Design review of the part built by this model. Coordinates are the model's own, in mm. A direction names the side the tool comes from. Round coordinates to 2 decimals unless told otherwise and drop trailing zeros. Loops run counter-clockwise (first coordinate to the right, second up) from the corner with the lowest first, then second, coordinate; pieces in that order, holes last. Notation, with made-up numbers: (60.5, 49) -> (99.5, 49) arc R19 cw to (99.5, 84) -> close; hole circle Ø11 at (52, 19). An arc over 180 degrees is marked (long way). Answer as CSV lines item,"result". Start each with the question number.
(1) Take a section at A-A, the plane z = -22.75. Write out the cut boundary in (x, y), and give its area (4 significant figures).
(2) For P1, Ø1.5, axis at x = 20.5, y = 1.5, coming from the -Z side; P2, Ø4, axis at x = 0, z = -4.5, coming from the +Y side; P3, Ø1, axis at y = 1.5, z = -71.5, coming from the -X side; P4, Ø0.6, axis at y = 1, z = -71, coming from the +X side, all flat-tipped, find the tip position at first contact; note any pin that passes through.
(3) Machinability: for faces 4 (the face through (21, 2, -70.5)), 5 (the face through (-10, 2, -2)), 6 (the face through (3.671, 1.521, -30.498)), 7 (the face through (-10, 2, -71)), which of the approach directions +Z, -Z, +X, -X, +Y, -Y give a long, thin tool a straight path to every point of the face, cutting with its end or side? Answer none if there is none.
(4) Take a section at D-D, the plane y = 2.45. State how many separate pieces and enclosed holes the cut face has, and give its area (3 significant figures).
(5) Take a section at C-C, the plane z = -36.75. Write out the cut boundary in (x, y).
(6) Take a section at B-B, the plane x = -28.5. Write out the cut boundary in (y, z).
(7) Draft analysis for pull direction X (two halves, no side actions). For faces 1 (the face through (10, 2, -2)), 2 (the face through (0.222, 1.521, -41.795)), 3 (the face through (21, 2, -3)), state which applies: +X half, -X half, draft (parallel to the pull), parting line (faces both ways), or undercut.
(8) To check wall thickness, follow line 1 (X direction, y = 1.15, z = -36.75); line 2 (X direction, y = 0.5, z = -41); line 3 (X direction, y = 2.2, z = -22.75). State the ranges of each line that lie inside material, in increasing order. Write a range as from..to.
from build123d import *

# Parameters (mm, degrees)
BOSS_EXTRUDE1_DEPTH   = 3
CROQUIS13_W           = 23
CROQUIS13_H           = 3
CORTAR_EXTRUIR3_DEPTH = 81.624127902
CUT_EXTRUDE1_REACH    = 82.624
SKETCH3_R             = 1.2
SKETCH3_R_2           = 5.05
SKETCH3_R_3           = 1.75
CHAFL_N3_SIZE         = 1
CORTAR_EXTRUIR2_DEPTH = 81.624127902


with BuildPart() as part:
    # Sketch1 → Boss-Extrude1 (new body)
    with BuildSketch(Plane(origin=(0, 0, 0), x_dir=(1, 0, 0), z_dir=(0, 1, 0))):
        Polygon((-33, 27.237606732), (-33, 0), (33, 0), (33, 73.5), (-33, 73.5), align=None)
    extrude(amount=BOSS_EXTRUDE1_DEPTH)

    # Croquis13 → Cortar-Extruir3 (cut, through all)
    with BuildSketch(Plane(origin=(0, 3, 0), x_dir=(1, 0, 0), z_dir=(0, 1, 0))):
        with Locations((-21.5, 72)):
            Rectangle(CROQUIS13_W, CROQUIS13_H)
        with Locations((21.5, 72)):
            Rectangle(CROQUIS13_W, CROQUIS13_H)
        with Locations((-21.5, 1.5)):
            Rectangle(CROQUIS13_W, CROQUIS13_H)
        with Locations((21.5, 1.5)):
            Rectangle(CROQUIS13_W, CROQUIS13_H)
    extrude(amount=-CORTAR_EXTRUIR3_DEPTH, mode=Mode.SUBTRACT)

    # Sketch3 → Cut-Extrude1 (cut, up to next)
    with BuildSketch(Plane(origin=(0, 3, 0), x_dir=(1, 0, 0), z_dir=(0, 1, 0)), mode=Mode.PRIVATE) as cut_extrude1_sk1:
        with Locations(Location((-20.9, 13.25, 0), (0, 0, 270))):
            Circle(SKETCH3_R)
    cut_extrude1_tool1 = extrude(cut_extrude1_sk1.sketch, amount=-CUT_EXTRUDE1_REACH, mode=Mode.PRIVATE) & part.part
    # Sketch3 → Cut-Extrude1 (cut, up to next)
    with BuildSketch(Plane(origin=(0, 3, 0), x_dir=(1, 0, 0), z_dir=(0, 1, 0)), mode=Mode.PRIVATE) as cut_extrude1_sk2:
        with Locations(Location((0, 36.75, 0), (0, 0, 270))):
            Circle(SKETCH3_R_2)
    cut_extrude1_tool2 = extrude(cut_extrude1_sk2.sketch, amount=-CUT_EXTRUDE1_REACH, mode=Mode.PRIVATE) & part.part
    # Sketch3 → Cut-Extrude1 (cut, up to next)
    with BuildSketch(Plane(origin=(0, 3, 0), x_dir=(1, 0, 0), z_dir=(0, 1, 0)), mode=Mode.PRIVATE) as cut_extrude1_sk3:
        with Locations(Location((-16.9, 49.75, 0), (0, 0, 270))):
            Circle(SKETCH3_R)
    cut_extrude1_tool3 = extrude(cut_extrude1_sk3.sketch, amount=-CUT_EXTRUDE1_REACH, mode=Mode.PRIVATE) & part.part
    # Sketch3 → Cut-Extrude1 (cut, up to next)
    with BuildSketch(Plane(origin=(0, 3, 0), x_dir=(1, 0, 0), z_dir=(0, 1, 0)), mode=Mode.PRIVATE) as cut_extrude1_sk4:
        with Locations(Location((25.6, 36.75, 0), (0, 0, 270))):
            Circle(SKETCH3_R)
    cut_extrude1_tool4 = extrude(cut_extrude1_sk4.sketch, amount=-CUT_EXTRUDE1_REACH, mode=Mode.PRIVATE) & part.part
    # Sketch3 → Cut-Extrude1 (cut, up to next)
    with BuildSketch(Plane(origin=(0, 3, 0), x_dir=(1, 0, 0), z_dir=(0, 1, 0)), mode=Mode.PRIVATE) as cut_extrude1_sk5:
        with Locations(Location((0, 4.5, 0), (0, 0, 270))):
            Circle(SKETCH3_R_3)
    cut_extrude1_tool5 = extrude(cut_extrude1_sk5.sketch, amount=-CUT_EXTRUDE1_REACH, mode=Mode.PRIVATE) & part.part
    # Sketch3 → Cut-Extrude1 (cut, up to next)
    with BuildSketch(Plane(origin=(0, 3, 0), x_dir=(1, 0, 0), z_dir=(0, 1, 0)), mode=Mode.PRIVATE) as cut_extrude1_sk6:
        with Locations(Location((0, 69, 0), (0, 0, 270))):
            Circle(SKETCH3_R_3)
    cut_extrude1_tool6 = extrude(cut_extrude1_sk6.sketch, amount=-CUT_EXTRUDE1_REACH, mode=Mode.PRIVATE) & part.part
    # Sketch3 → Cut-Extrude1 (cut, up to next)
    with BuildSketch(Plane(origin=(0, 3, 0), x_dir=(1, 0, 0), z_dir=(0, 1, 0)), mode=Mode.PRIVATE) as cut_extrude1_sk7:
        with Locations(Location((-28.5, 22.75, 0), (0, 0, 270))):
            Circle(SKETCH3_R_3)
    cut_extrude1_tool7 = extrude(cut_extrude1_sk7.sketch, amount=-CUT_EXTRUDE1_REACH, mode=Mode.PRIVATE) & part.part
    add(cut_extrude1_tool1.solids().sort_by_distance((-20.9, 3, -13.25))[0], mode=Mode.SUBTRACT)
    add(cut_extrude1_tool2.solids().sort_by_distance((0, 3, -36.75))[0], mode=Mode.SUBTRACT)
    add(cut_extrude1_tool3.solids().sort_by_distance((-16.9, 3, -49.75))[0], mode=Mode.SUBTRACT)
    add(cut_extrude1_tool4.solids().sort_by_distance((25.6, 3, -36.75))[0], mode=Mode.SUBTRACT)
    add(cut_extrude1_tool5.solids().sort_by_distance((0, 3, -4.5))[0], mode=Mode.SUBTRACT)
    add(cut_extrude1_tool6.solids().sort_by_distance((0, 3, -69))[0], mode=Mode.SUBTRACT)
    add(cut_extrude1_tool7.solids().sort_by_distance((-28.5, 3, -22.75))[0], mode=Mode.SUBTRACT)

    # Chaflán3
    chafl_n3_edges = [part.edges().sort_by_distance(p)[0] for p in [
        (-33, 1.5, -70.5),
        (-10, 1.5, -73.5),
        (33, 1.5, -70.5),
        (10, 1.5, -73.5),
        (-33, 1.5, -3),
        (-10, 1.5, 0),
        (33, 1.5, -3),
        (10, 1.5, 0),
    ]]
    chamfer(chafl_n3_edges, length=CHAFL_N3_SIZE)

    # Croquis12 → Cortar-Extruir2 (cut, through all)
    with BuildSketch(Plane(origin=(0, 3, 0), x_dir=(1, 0, 0), z_dir=(0, 1, 0))):
        with BuildLine():
            ThreePointArc((-9.309773091, 42.125), (-10.75, 36.75), (-9.309773091, 31.375))
            ThreePointArc((-9.309773091, 31.375), (-6.919228634, 30.734455543), (-6.278684177, 33.125))
            ThreePointArc((-6.278684177, 33.125), (-7.25, 36.75), (-6.278684177, 40.375))
            ThreePointArc((-6.278684177, 40.375), (-6.919228634, 42.765544457), (-9.309773091, 42.125))
        make_face()
        with BuildLine():
            ThreePointArc((9.309773091, 42.125), (5.375, 46.059773091), (0, 47.5))
            ThreePointArc((0, 47.5), (-1.75, 45.75), (0, 44))
            ThreePointArc((0, 44), (3.625, 43.028684177), (6.278684177, 40.375))
            ThreePointArc((6.278684177, 40.375), (8.669228634, 39.734455543), (9.309773091, 42.125))
        make_face()
        with BuildLine():
            ThreePointArc((0, 26), (5.375, 27.440226909), (9.309773091, 31.375))
            ThreePointArc((9.309773091, 31.375), (8.669228634, 33.765544457), (6.278684177, 33.125))
            ThreePointArc((6.278684177, 33.125), (3.625, 30.471315823), (0, 29.5))
            ThreePointArc((0, 29.5), (-1.75, 27.75), (0, 26))
        make_face()
    extrude(amount=-CORTAR_EXTRUIR2_DEPTH, mode=Mode.SUBTRACT)


solid = part.part
The answers:
1,outline,"(-33, 0) -> (-30.25, 0) -> (-30.25, 3) -> (-33, 3) -> close; (-26.75, 0) -> (33, 0) -> (33, 3) -> (-26.75, 3) -> close"
1,area,"187.5 mm²"
2,P1,"z = -70.5"
2,P2,"y = 3"
2,P3,"x = -10"
2,P4,"x = 10"
3,face 4,"-Z, +X, +Y, -Y"
3,face 5,"+Z, -X, +Y, -Y"
3,face 6,"+Y, -Y"
3,face 7,"-Z, -X, +Y, -Y"
4,separate pieces,"1"
4,enclosed holes,"10"
4,area,"4,320 mm²"
5,outline,"(-33, 0) -> (-10.75, 0) -> (-10.75, 3) -> (-33, 3) -> close; (-7.25, 0) -> (-5.05, 0) -> (-5.05, 3) -> (-7.25, 3) -> close; (5.05, 0) -> (24.4, 0) -> (24.4, 3) -> (5.05, 3) -> close; (26.8, 0) -> (33, 0) -> (33, 3) -> (26.8, 3) -> close"
6,outline,"(0, -70.5) -> (3, -70.5) -> (3, -24.5) -> (0, -24.5) -> close; (0, -21) -> (3, -21) -> (3, -3) -> (0, -3) -> close"
7,face 1,"+X half"
7,face 2,"undercut"
7,face 3,"draft"
8,line 1,"-33..-10.75, -7.25..-5.05, 5.05..24.4, 26.8..33"
8,line 2,"-33..-9.87, -6.06..-2.73, 2.73..5.87, 9.53..33"
8,line 3,"-33..-30.25, -26.75..33"
